from build123d import *

# Parameters (mm, degrees)
SKETCH1_W                               = 100
SKETCH1_H                               = 40
BASE_PLATE_DEPTH                        = 10
VERT_BOSS_DEPTH                         = 10
SKETCH5_W                               = 40
SKETCH5_H                               = 3
SLOT_DEPTH                              = 121.933866224
HOLE_WIZARD_7_0_7_1_D                   = 7
CBORE_FOR_M8_HEX_HEAD_BOLT1_D           = 9
CBORE_FOR_M8_HEX_HEAD_BOLT1_CBORE_D     = 18.01
CBORE_FOR_M8_HEX_HEAD_BOLT1_CBORE_DEPTH = 5.68
FILLET_1_R                              = 6
FILLET_2_R                              = 3


with BuildPart() as part:
    # Sketch1 → Base Plate (new body)
    with BuildSketch(Plane(origin=(0, 0, 0), x_dir=(1, 0, 0), z_dir=(0, 1, 0))):
        with Locations((50, 20)):
            Rectangle(SKETCH1_W, SKETCH1_H)
    extrude(amount=BASE_PLATE_DEPTH)

    # Sketch2 → Vert Boss (add)
    with BuildSketch(Plane.XY):
        with BuildLine():
            Line((30, 0), (30, 35))
            ThreePointArc((30, 35), (50, 55), (70, 35))
            Line((70, 35), (70, 0))
            Line((70, 0), (30, 0))
        make_face()
    extrude(amount=-VERT_BOSS_DEPTH)

    # Sketch5 → Slot (cut, through all)
    with BuildSketch(Plane.XY):
        with Locations((50, 1.5)):
            Rectangle(SKETCH5_W, SKETCH5_H)
    extrude(amount=-SLOT_DEPTH, mode=Mode.SUBTRACT)

    # Ø7.0 (7) 直徑孔1 (through all)
    with Locations(Plane(origin=(0, 10, 0), x_dir=(-1, 0, 0), z_dir=(0, 1, 0))):
        with Locations((-88, -28), (-12, -28)):
            Hole(HOLE_WIZARD_7_0_7_1_D / 2)

    # CBORE for M8 Hex Head Bolt1 (through all)
    with Locations(Plane.XY):
        with Locations((50, 35)):
            CounterBoreHole(CBORE_FOR_M8_HEX_HEAD_BOLT1_D / 2, CBORE_FOR_M8_HEX_HEAD_BOLT1_CBORE_D / 2, CBORE_FOR_M8_HEX_HEAD_BOLT1_CBORE_DEPTH)

    # 圓角1
    # the kernel refuses this fillet: 6 mm, written as the material it adds along each edge
    with BuildSketch(Plane(origin=(70, 3, 0), x_dir=(-1, 0, 0), z_dir=(0, 0, -1))) as fillet_1_piece_1:
        with BuildLine():
            CenterArc((5.196152423, -6), FILLET_1_R, 90, 60)
            Line((0, -3), (0, 0))
            Line((0, 0), (5.196152423, 0))
        make_face()
    extrude(amount=40)
    with BuildSketch(Plane(origin=(30, 3, 0), x_dir=(0, -1, 0), z_dir=(0, 0, -1))) as fillet_1_piece_2:
        with BuildLine():
            CenterArc((6, -5.196152423), FILLET_1_R, 120, 60)
            Line((0, -5.196152423), (0, 0))
            Line((0, 0), (3, 0))
        make_face()
    extrude(amount=40)
    # the kernel refuses this fillet: 6 mm, written as the material it takes off along each edge
    with BuildSketch(Plane(origin=(0, -15, 0), x_dir=(1, 0, 0), z_dir=(0, 1, 0)), Plane(origin=(0, -15, -40), x_dir=(0, 0, 1), z_dir=(0, 1, 0))) as fillet_1_2_piece_1:
        with BuildLine():
            CenterArc((FILLET_1_R, FILLET_1_R), FILLET_1_R, 180, 90)
            Line((0, FILLET_1_R), (0, 0))
            Line((0, 0), (FILLET_1_R, 0))
        make_face()
    extrude(amount=40, mode=Mode.SUBTRACT)
    with BuildSketch(Plane(origin=(100, -15, -40), x_dir=(0, 0, 1), z_dir=(0, 1, 0)), Plane(origin=(100, -15, 0), x_dir=(-1, 0, 0), z_dir=(0, 1, 0))) as fillet_1_2_piece_2:
        with BuildLine():
            CenterArc((FILLET_1_R, -FILLET_1_R), FILLET_1_R, 90, 90)
            Line((0, -FILLET_1_R), (0, 0))
            Line((0, 0), (FILLET_1_R, 0))
        make_face()
    extrude(amount=40, mode=Mode.SUBTRACT)

    # 圓角2
    fillet_2_edges = [part.edges().sort_by_distance(p)[0] for p in [
        (82, 10, 0),
        (30, 22.5, -10),
        (70, 22.5, -10),
        (30, 22.5, 0),
        (70, 22.5, 0),
        (50, 55, 0),
        (30, 10, -5),
        (50, 55, -10),
        (70, 10, -5),
        (50, 10, -10),
        (18, 10, 0),
        (0, 10, -20),
        (100, 10, -20),
        (50, 10, -40),
        (98.242640687, 10, -1.757359313),
        (98.242640687, 10, -38.242640687),
        (1.757359313, 10, -38.242640687),
        (1.757359313, 10, -1.757359313),
    ]]
    fillet(fillet_2_edges, radius=FILLET_2_R)


solid = part.part
Source: CAD feature listing. Evaluate the final solid. Frame: model axes, mm. A direction names the side the tool comes from. Coordinates: 2 decimals unless noted, no trailing zeros. Loops run counter-clockwise (first coordinate to the right, second up) from the corner with the lowest first, then second, coordinate; pieces in that order, holes last. Notation, with made-up numbers: (52.25, 33) - (107.25, 33) arc R17 ccw to (107.25, 61) - close; hole circle Ø4 at (18, 49.25). An arc over 180 degrees is marked (long way). One line per item, written item: value. Start each with the question number.
1. Set-up query: faces 1 (the flat face through (30, 24, -5)), 2 (the cylindrical face through (83.65, 9.1, -0.86)), 3 (the cylindrical face through (30.9, 24.15, -0.86)). Return all of +Z, -Z, +X, -X, +Y, -Y with unobstructed straight access to the full face (end or side cutting, diameter ignored); none if empty.
2. Section D-D (y = 16). Return the cut outline in (x, z), and give its area (3 significant figures).
3. Section A-A (z = -28). Return the cut outline in (x, y), and give its area (3 significant figures).
4. Section C-C (y = 32.5). Return the cut outline in (x, z), and give its area (3 significant figures).
5. Section B-B (x = 50). Return the cut outline in (y, z) (3 decimals), and give its area (3 significant figures).
6. Ray query, L1, parallel to Z at x = 12, y = 4; L2, parallel to Y at x = 82, z = -3; L3, parallel to Y at x = 54.5, z = -33.5. Return the intervals inside material, ascending.
7. Mould query, pull axis Z, two halves, no side actions, for faces 4 (the cylindrical face through (67.8, 2.2, -19.7)), 5 (the cylindrical face through (91.34, 4.93, -26.95)), 6 (the cylindrical face through (30.86, 24.15, -9.1)). Classes: pulls with the +Z half, pulls with the -Z half, needs draft (parallel to the pull), parting line crosses it, or undercut.
8. Contact query for flat-ended pins moving along their axis: P1, Ø6, axis at x = 66.5, y = 23.5, coming from the -Z side; P2, Ø4, axis at x = 55.5, y = 40, coming from the +Z side; P3, Ø6.5, axis at x = 88, z = -28, coming from the -Y side; P4, Ø23.5, axis at x = 45.5, z = -23.5, coming from the -Y side. Output: stop coordinate, or through.
Verdict:
1. face 1: +Z, -Z, -X, +Y
1. face 2: +Z, +X, +Y
1. face 3: +Z, -X, +Y
2. outline: (30, -7) arc R3 ccw to (33, -10) - (67, -10) arc R3 ccw to (70, -7) - (70, -3) arc R3 ccw to (67, 0) - (33, 0) arc R3 ccw to (30, -3) - close
2. area: 392 mm2
3. outline: (0, 0) - (8.5, 0) - (8.5, 10) - (3, 10) arc R3 ccw to (0, 7) - close; (15.5, 0) - (30, 0) arc R6 cw to (35.2, 3) - (64.8, 3) arc R6 cw to (70, 0) - (84.5, 0) - (84.5, 10) - (15.5, 10) - close; (91.5, 0) - (100, 0) - (100, 7) arc R3 ccw to (97, 10) - (91.5, 10) - close
3. area: 745 mm2
4. outline: (30, -7) arc R3 ccw to (33, -10) - (46.26, -10) - (46.26, -5.68) - (41.35, -5.68) - (41.35, 0) - (33, 0) arc R3 ccw to (30, -3) - close; (53.74, -10) - (67, -10) arc R3 ccw to (70, -7) - (70, -3) arc R3 ccw to (67, 0) - (58.65, 0) - (58.65, -5.68) - (53.74, -5.68) - close
4. area: 262 mm2
5. outline: (3, -40) - (7, -40) arc R3 ccw to (10, -37) - (10, -13) arc R3 cw to (13, -10) - (30.5, -10) - (30.5, -5.68) - (25.995, -5.68) - (25.995, 0) - (3, 0) - close; (39.5, -10) - (52, -10) arc R3 ccw to (55, -7) - (55, -3) arc R3 ccw to (52, 0) - (44.005, 0) - (44.005, -5.68) - (39.5, -5.68) - close
5. area: 585 mm2
6. L1: z = -40 to -31.5, -24.5 to 0
6. L2: y = 0 to 10
6. L3: y = 3 to 10
7. face 4: needs draft
7. face 5: undercut
7. face 6: pulls with the -Z half
8. P1: stops at z = -10
8. P2: stops at z = 0
8. P3: passes through
8. P4: stops at y = 2.82
